Study the drawing (mm; zero at the part's minimum x, y, z) and answer. A direction names the side the tool comes from. Coordinates: 2 decimals unless noted, no trailing zeros. Order: outer loops, then holes, each group sorted by start corner. A loop starts at its lowest first (then second) coordinate and runs counter-clockwise, first axis right, second up. Notation, with made-up numbers: (18.5, -9) -> (32.5, -9) arc R16 cw to (32.5, 4) -> close; hole circle Ø8 at (-32.75, -9). An arc over 180 degrees is marked (long way). Put each result on its own line as item: value. Start each with the question number.
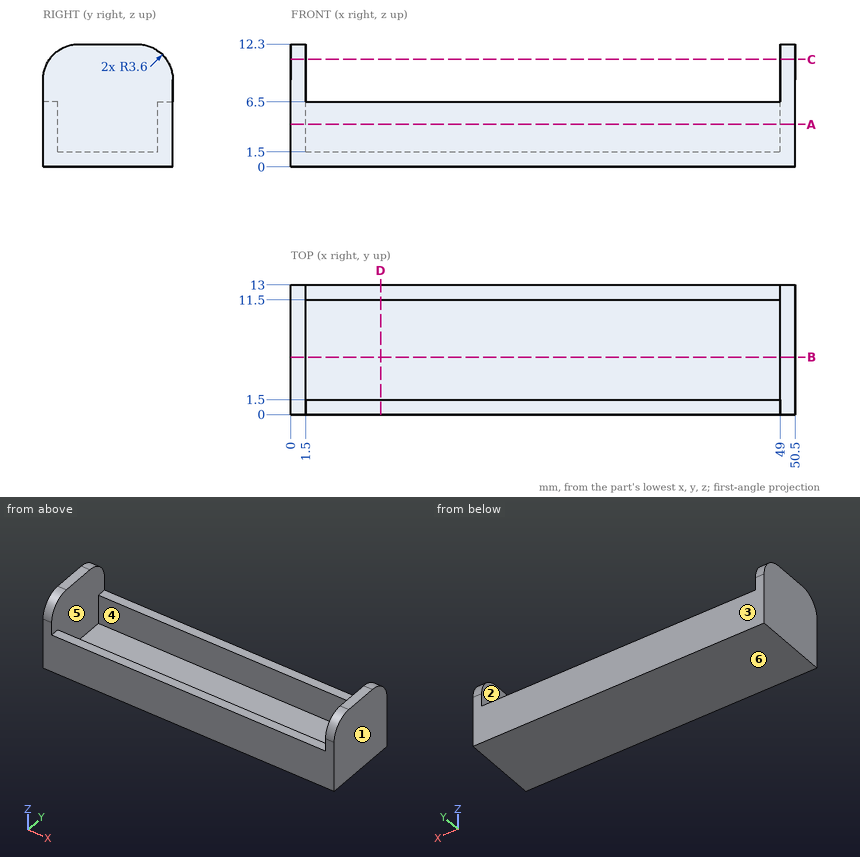
(1) For a pull along Y with two mould halves and no side action, classify the marked faces 1, 2, 3 and 4 as released by +Y, released by -Y, zero draft, split by the parting line, or undercut.
(2) Each of these flat-tipped pins is pushed along its axis until it touches: P1, Ø1.2, axis at x = 29, y = 0.5, coming from the +Z side; P2, Ø3, axis at x = 34, y = 4.5, coming from the +Z side; P3, Ø1.5, axis at x = 41.5, z = 7.5, coming from the +Y side; P4, Ø6, axis at y = 8, z = 10.5, coming from the -X side. Where does it stop, or does it pass through?
(3) The part is cut by section B-B on y = 5.75. Determine the outline of the cut face in (x, z), plus the area to 3 significant figures.
(4) The part is cut by section D-D on x = 9. Determine the outline of the cut face in (y, z), plus the area to 3 significant figures.
(5) The part is cut by section A-A on z = 4.25. Determine the outline of the cut face in (x, y), plus the area to 4 significant figures.
(6) A tool of negligible diameter and unlimited length cuts with its end or side. For the marked faces 5 and 6, from which of +Z, -Z, +X, -X, +Y, -Y can it reach the whole face along a straight path? Write none if from no direction.
(7) Find the intervals of material crossed by L1, parallel to Y at x = 45, z = 6; L2, parallel to X at y = 6, z = 7.25; L3, parallel to Z at x = 22, y = 7.25, in increasing order.
(8) The part is cut by section C-C on z = 10.75. Determine the outline of the cut face in (x, y).
Worked out:
1. face 1: zero draft
1. face 2: undercut
1. face 3: released by +Y
1. face 4: undercut
2. P1: z = 6.5
2. P2: z = 1.5
2. P3: through
2. P4: x = 0
3. outline: (0, 0) -> (50.5, 0) -> (50.5, 12.3) -> (49, 12.3) -> (49, 1.5) -> (1.5, 1.5) -> (1.5, 12.3) -> (0, 12.3) -> close
3. area: 108 mm2
4. outline: (0, 0) -> (13, 0) -> (13, 6.5) -> (11.5, 6.5) -> (11.5, 1.5) -> (1.5, 1.5) -> (1.5, 6.5) -> (0, 6.5) -> close
4. area: 34.5 mm2
5. outline: (0, 0) -> (50.5, 0) -> (50.5, 13) -> (0, 13) -> close; hole (1.5, 1.5) -> (49, 1.5) -> (49, 11.5) -> (1.5, 11.5) -> close
5. area: 181.5 mm2
6. face 5: +Z
6. face 6: -Z, +X, -X, +Y, -Y
7. L1: 0 to 1.5, 11.5 to 13
7. L2: 0 to 1.5, 49 to 50.5
7. L3: 0 to 1.5
8. outline: (0, 0.64) -> (1.5, 0.64) -> (1.5, 12.36) -> (0, 12.36) -> close; (49, 0.64) -> (50.5, 0.64) -> (50.5, 12.36) -> (49, 12.36) -> close
